from build123d import *

# Parameters (mm, degrees)
SKETCH1_W           = 150.33165829
SKETCH1_H           = 100
BOSS_EXTRUDE1_DEPTH = 10
SKETCH2_W           = 14.278709015
SKETCH2_H           = 9.735554689
SKETCH2_W_2         = 30.342256657
SKETCH2_H_2         = 20.971853865
SKETCH2_W_3         = 41.051288419
SKETCH2_H_3         = 22.198930422
CUT_EXTRUDE1_DEPTH  = 5


with BuildPart() as part:
    # Sketch1 → Boss-Extrude1 (new body)
    with BuildSketch(Plane.XY):
        with Locations((30.442211055, -24.120603015)):
            Rectangle(SKETCH1_W, SKETCH1_H)
    extrude(amount=BOSS_EXTRUDE1_DEPTH)

    # Sketch2 → Cut-Extrude1 (cut)
    with BuildSketch(Plane.XY.offset(10)):
        with Locations((-25.333996036, 4.867777345)):
            Rectangle(SKETCH2_W, SKETCH2_H)
        with Locations((56.210818731, -21.945330938)):
            Rectangle(SKETCH2_W_2, SKETCH2_H_2)
        with Locations((6.793099248, -50.000763105)):
            Rectangle(SKETCH2_W_3, SKETCH2_H_3)
    extrude(amount=-CUT_EXTRUDE1_DEPTH, mode=Mode.SUBTRACT)


solid = part.part
For this review, take the finished solid that the model builds, in its own axes (mm). A direction names the side the tool comes from. Give positions to 0.01 mm unless a question says otherwise; leave off trailing zeros. Order: outer loops, then holes, each group sorted by start corner. A loop starts at its lowest first (then second) coordinate and runs counter-clockwise, first axis right, second up. Notation, with made-up numbers: M 81,27 L 108,27 A28 cw 108,52 Z; hole C 15,57 d7. An arc over 180 degrees is marked long. Answer in a Markdown table with one row per item. Add a question column.
(1) Mouldability with a two-part tool opening along Y and no side actions: class faces 3 (the face through (-44.724, -25, 5)), 4 (the face through (7, -38.901, 8)), 5 (the face through (29, 25.879, 5)) as +Y half, -Y half, draft (parallel to the pull), parting line (faces both ways), or undercut.
(2) Consider section B-B on y = -20.5. State the section outline as (x, z) points.
(3) For faces 1 (the face through (-25, 0, 8)), 2 (the face through (105.608, -25, 5)), list the 3-axis set-ups (+Z, -Z, +X, -X, +Y, -Y) from which the entire face can be reached by the end or side of a thin tool; tool diameter is ignored.
(4) Consider section A-A on x = -30.5. State the section outline as (y, z) points, and give its area (3 significant figures).
(5) Wall thickness on probe 1 along Y at (x, z) = (44.5, 8.75); probe 2 along Y at (x, z) = (-21.5, 8.75); probe 3 along X at (y, z) = (-26, 7.75): over which ranges is each line inside the solid? List them lowest first. Write a range as [from, to].
(6) For pin 1 (10.5 mm diameter, centred on x = 53.5, y = -20, fed in from +Z), flat-tipped, find the tip position at first contact; note if it passes through.
Evaluation:
| question | item | result |
|---|---|---|
| 1 | face 3 | draft |
| 1 | face 4 | undercut |
| 1 | face 5 | +Y half |
| 2 | outline | M -44.72,0 L 105.61,0 L 105.61,10 L 71.38,10 L 71.38,5 L 41.04,5 L 41.04,10 L -44.72,10 Z |
| 3 | face 1 | +Z |
| 3 | face 2 | +Z, -Z, +X, +Y, -Y |
| 4 | outline | M -74.12,0 L 25.88,0 L 25.88,10 L 9.74,10 L 9.74,5 L 0,5 L 0,10 L -74.12,10 Z |
| 4 | area | 951 mm^2 |
| 5 | probe 1 | y = [-74.12, -32.43], [-11.46, 25.88] |
| 5 | probe 2 | y = [-74.12, 0], [9.74, 25.88] |
| 5 | probe 3 | x = [-44.72, 41.04], [71.38, 105.61] |
| 6 | pin 1 | stops at z = 5 |
